The model under review builds one solid part; all positions refer to its coordinate system, in mm. A direction names the side the tool comes from. Coordinates: 2 decimals unless noted, no trailing zeros. Loops run counter-clockwise (first coordinate to the right, second up) from the corner with the lowest first, then second, coordinate; pieces in that order, holes last. Notation, with made-up numbers: M 34.5,66.5 L 64.5,66.5 A28 cw 64.5,92.5 Z; hole C -29,64.25 d6. An arc over 180 degrees is marked long. Use CSV: the item, a comma, the result in double quotes. Start each with the question number.
from build123d import *

# Parameters (mm, degrees)
BOSS_EXTRUDE1_DEPTH = 101.6
SKETCH2_R           = 6.54812
CUT_EXTRUDE1_DEPTH  = 304.8


with BuildPart() as part:
    # Sketch1 → Boss-Extrude1 (new body)
    with BuildSketch(Plane.XY):
        with BuildLine():
            Line((-76.777987096, 41.427423626), (102.292012904, 41.427423626))
            Line((102.292012904, 41.427423626), (102.292012904, 35.077423626))
            Line((102.292012904, 35.077423626), (-75.507987096, 35.077423626))
            ThreePointArc((-75.507987096, 35.077423626), (-89.87639689, 29.12583342), (-95.827987096, 14.757423626))
            Line((-95.827987096, 14.757423626), (-95.827987096, -41.122576374))
            Line((-95.827987096, -41.122576374), (-102.177987096, -41.122576374))
            Line((-102.177987096, -41.122576374), (-102.177987096, 16.027423626))
            ThreePointArc((-102.177987096, 16.027423626), (-94.738499338, 33.987935868), (-76.777987096, 41.427423626))
        make_face()
    extrude(amount=BOSS_EXTRUDE1_DEPTH)

    # Sketch2 → Cut-Extrude1 (cut)
    with BuildSketch(Plane.ZY.offset(102.177987096)):
        with Locations((25.4, -12.547576374)):
            Circle(SKETCH2_R)
        with Locations((76.2, -12.547576374)):
            Circle(SKETCH2_R)
    extrude(amount=-CUT_EXTRUDE1_DEPTH, mode=Mode.SUBTRACT)


solid = part.part
1. Add section D-D (y = -34.5). Write out the cut boundary in (x, z).
2. Add section B-B (z = 67). Write out the cut boundary in (x, y).
3. Add section A-A (z = 25.4). Write out the cut boundary in (x, y), plus the area to 3 significant figures.
4. To check wall thickness, follow line 1 along X through (y, z) = (-19, 28); line 2 along Y through (x, z) = (-99, 76.2); line 3 along Y through (x, z) = (-14.5, 77). State the ranges of each line that lie inside material, in increasing order.
5. Draft analysis for pull direction Y (two halves, no side actions). For faces 1 (the cylindrical face through (-99.047, -15.056, 82.249)), 2 (the cylindrical face through (-90, 29, 50)), 3 (the flat face through (-30, 37, 101.6)), state which applies: released by +Y, released by -Y, zero draft, split by the parting line, or undercut.
6. Add section C-C (x = -15). Write out the cut boundary in (y, z).
7. For faces 4 (the flat face through (-95.828, -13, 50)), 5 (the cylindrical face through (-99.047, -10.581, 31.646)), list the 3-axis set-ups (+Z, -Z, +X, -X, +Y, -Y) from which the entire face can be reached by the end or side of a thin tool; tool diameter is ignored.
8. Insertion check: pin 1 Ø12 at (x, z) = (-60, 72) entering from -Y; pin 2 Ø12 at (y, z) = (-12.55, 76.2) entering from -X; pin 3 Ø5 at (y, z) = (16, 59.5) entering from +X; pin 4 Ø12 at (y, z) = (-30.5, 26.5) entering from +X. Each pin has a flat end and moves straight along its axis. Give the tip position at first contact, or say it passes through.
Solved:
1,outline,"M -102.18,0 L -95.83,0 L -95.83,101.6 L -102.18,101.6 Z"
2,outline,"M -102.18,-41.12 L -95.83,-41.12 L -95.83,14.76 A20.32 cw -75.51,35.08 L 102.29,35.08 L 102.29,41.43 L -76.78,41.43 A25.4 ccw -102.18,16.03 Z"
3,outline,"M -102.18,-41.12 L -95.83,-41.12 L -95.83,-19.1 L -102.18,-19.1 Z; M -102.18,-6 L -95.83,-6 L -95.83,14.76 A20.32 cw -75.51,35.08 L 102.29,35.08 L 102.29,41.43 L -76.78,41.43 A25.4 ccw -102.18,16.03 Z"
3,area,"1,650 mm^2"
4,line 1,"x = -102.18 to -95.83"
4,line 2,"y = -41.12 to -19.1, -6 to 28.33"
4,line 3,"y = 35.08 to 41.43"
5,face 1,"undercut"
5,face 2,"released by -Y"
5,face 3,"zero draft"
6,outline,"M 35.08,0 L 41.43,0 L 41.43,101.6 L 35.08,101.6 Z"
7,face 4,"+Z, -Z, +X, -Y"
7,face 5,"+X, -X"
8,pin 1,"stops at y = 35.08"
8,pin 2,"passes through"
8,pin 3,"stops at x = -95.48"
8,pin 4,"stops at x = -95.83"
